from build123d import *

# Parameters (mm, degrees)
BOSS_EXTRUDE1_DEPTH = 3
SKETCH2_R           = 2
BOSS_EXTRUDE2_DEPTH = 1
SKETCH4_R           = 1.5
BOSS_EXTRUDE3_DEPTH = 61


with BuildPart() as part:
    # Sketch1 → Boss-Extrude1 (new body)
    with BuildSketch(Plane.XY):
        Polygon((-3.176229493, 1.382594015), (-2.785476286, -2.059398422), (0.390753207, -3.441992436), (3.176229493, -1.382594015), (2.785476286, 2.059398422), (-0.390753207, 3.441992436), align=None)
    extrude(amount=BOSS_EXTRUDE1_DEPTH)

    # Sketch2 → Boss-Extrude2 (add)
    with BuildSketch(Plane.XY):
        Circle(SKETCH2_R)
    extrude(amount=-BOSS_EXTRUDE2_DEPTH)

    # Sketch4 → Boss-Extrude3 (add)
    with BuildSketch(Plane(origin=(0, 0, -1), x_dir=(-1, 0, 0), z_dir=(0, 0, -1))):
        Circle(SKETCH4_R)
    extrude(amount=BOSS_EXTRUDE3_DEPTH)


solid = part.part
For this review, take the finished solid that the model builds, in its own axes (mm). A direction names the side the tool comes from. Round coordinates to 2 decimals unless told otherwise and drop trailing zeros. Order: outer loops, then holes, each group sorted by start corner. A loop starts at its lowest first (then second) coordinate and runs counter-clockwise, first axis right, second up. Notation, with made-up numbers: M -39.75,-26 L 12.25,-26 A31 ccw 12.25,3 Z; hole C 64.5,-23 d11. An arc over 180 degrees is marked long. Use a Markdown table: item, result. Add a question column.
Item 1: Tool access review of faces 1 (the flat face through (1, 2, 0)), 2 (the flat face through (1.8, -2.4, 1.5)): name each direction out of +Z, -Z, +X, -X, +Y, -Y from which nothing blocks a thin tool from reaching the whole face with its end or side.
Item 2: To check wall thickness, follow line 1 along Z through (x, y) = (-1.75, 0.5); line 2 along Z through (x, y) = (2.5, 1.75); line 3 along Y through (x, z) = (0, -4). State the ranges of each line that lie inside material, in increasing order.
Item 3: Add section A-A, the plane y = -0.75. Give the boundary of the cut face in (x, z).
Item 4: Insertion check: pin 1 (2 mm diameter, centred on x = 0, z = -11, fed in from +Y); pin 2 (2 mm diameter, centred on x = 0.5, y = -2.5, fed in from -Z). Each pin has a flat end and moves straight along its axis. Give the tip position at first contact, or say it passes through.
Item 5: Add section B-B, the plane z = -25. Give the boundary of the cut face in (x, y).
Geometry results:
| question | item | result |
|---|---|---|
| 1 | face 1 | -Z |
| 1 | face 2 | +Z, -Z, +X, -Y |
| 2 | line 1 | z = -1 to 3 |
| 2 | line 2 | z = 0 to 3 |
| 2 | line 3 | y = -1.5 to 1.5 |
| 3 | outline | M -2.93,0 L -1.85,0 L -1.85,-1 L -1.3,-1 L -1.3,-62 L 1.3,-62 L 1.3,-1 L 1.85,-1 L 1.85,0 L 3.1,0 L 3.1,3 L -2.93,3 Z |
| 4 | pin 1 | stops at y = 1.5 |
| 4 | pin 2 | stops at z = -1 |
| 5 | outline | C 0,0 d3 |
